Can you work these out from the drawing? Everything is in mm from the part's minimum corner. A direction names the side the tool comes from. Coordinates: 2 decimals unless noted, no trailing zeros. Order: outer loops, then holes, each group sorted by start corner. A loop starts at its lowest first (then second) coordinate and runs counter-clockwise, first axis right, second up. Notation, with made-up numbers: (-13.5, 10) - (15.5, 10) arc R24 ccw to (15.5, 21) - close; hole circle Ø7 at (13.5, 10). An arc over 180 degrees is marked (long way). Answer as CSV lines item,"result". Start each with the question number.
Item 1: On a 3-axis mill with a long thin cutter (end or side, diameter ignored), from which of +Z, -Z, +X, -X, +Y, -Y can I reach the whole of each face in a straight line? I mean the marked faces 5, 6 and 7. Say none if no direction works.
Item 2: Imagine slicing it at C-C on x = 5.25. List the corners of the cut face in (y, z) for me.
Item 3: I'm going to push flat-ended pins straight in: pin 1 (1 mm diameter, centred on x = 12.5, z = 7.5, fed in from -Y); pin 2 (0.8 mm diameter, centred on x = 5.5, z = 3.5, fed in from +Y); pin 3 (4 mm diameter, centred on x = 7.5, y = 12, fed in from +Z). Where does each tip first touch, or does it pass through?
Item 4: I need wall thicknesses on line 1 (Z direction, x = 5.25, y = 18.75); line 2 (Y direction, x = 10, z = 2.25); line 3 (Z direction, x = 6.25, y = 4). Which ranges of each line are inside material? Lowest first, please.
Item 5: We'd pull the mould along Z, two halves only. Please class the marked faces 1, 2, 3 and 4: pulls with the +Z half, pulls with the -Z half, needs draft (parallel to the pull), parting line crosses it, or undercut.
Item 6: Imagine slicing it at A-A on z = 5.5. List the corners of the cut face in (x, y) for me.
Item 7: Imagine slicing it at D-D on y = 16.5. List the corners of the cut face in (x, z) for me.
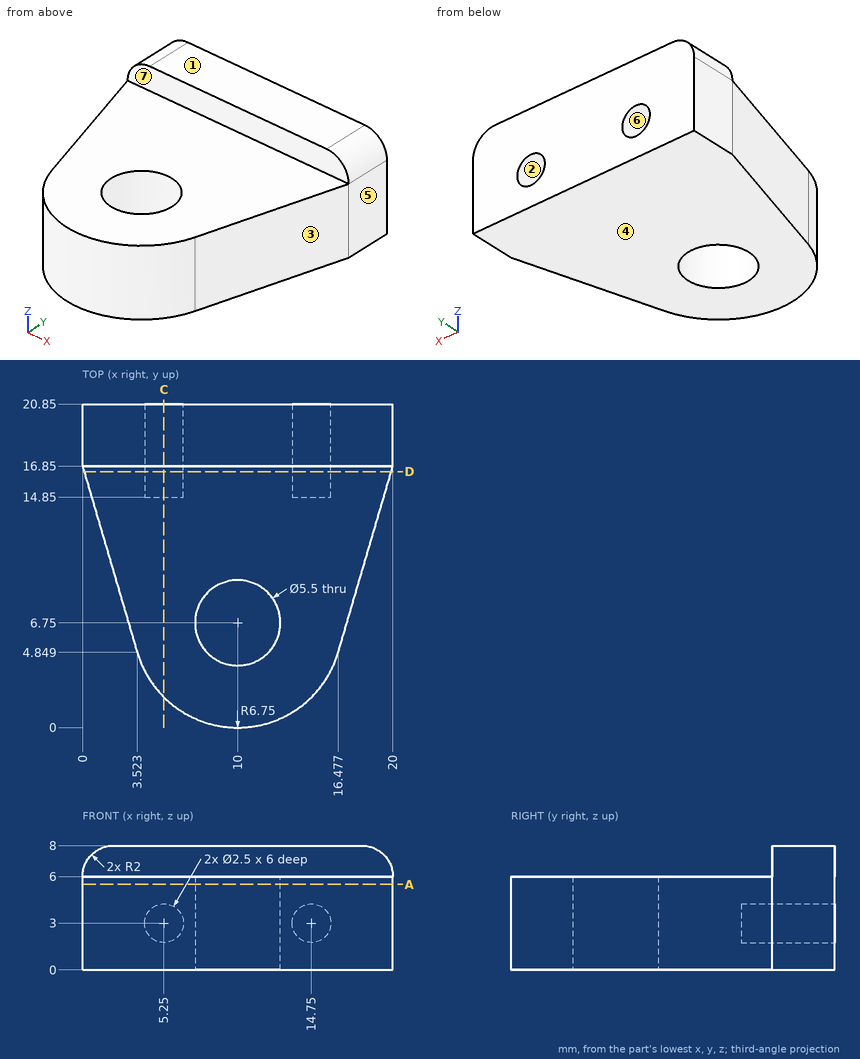
Responses:
1,face 5,"+Z, -Z, +X, +Y, -Y"
1,face 6,"+Y"
1,face 7,"+Z, +X, -X, -Y"
2,outline,"(1.95, 0) - (20.85, 0) - (20.85, 1.75) - (14.85, 1.75) - (14.85, 4.25) - (20.85, 4.25) - (20.85, 8) - (16.85, 8) - (16.85, 6) - (1.95, 6) - close"
3,pin 1,"stops at y = 16.85"
3,pin 2,"stops at y = 14.85"
3,pin 3,"stops at z = 6"
4,line 1,"z = 0 to 1.75, 4.25 to 8"
4,line 2,"y = 0 to 4, 9.5 to 20.85"
4,line 3,"z = 0 to 6"
5,face 1,"pulls with the +Z half"
5,face 2,"undercut"
5,face 3,"needs draft"
5,face 4,"pulls with the -Z half"
6,outline,"(0, 16.85) - (3.52, 4.85) arc R6.75 ccw to (16.48, 4.85) - (20, 16.85) - (20, 20.85) - (0, 20.85) - close; hole circle Ø5.5 at (10, 6.75)"
7,outline,"(0.1, 0) - (19.9, 0) - (19.9, 6) - (0.1, 6) - close; hole circle Ø2.5 at (5.25, 3); hole circle Ø2.5 at (14.75, 3)"
